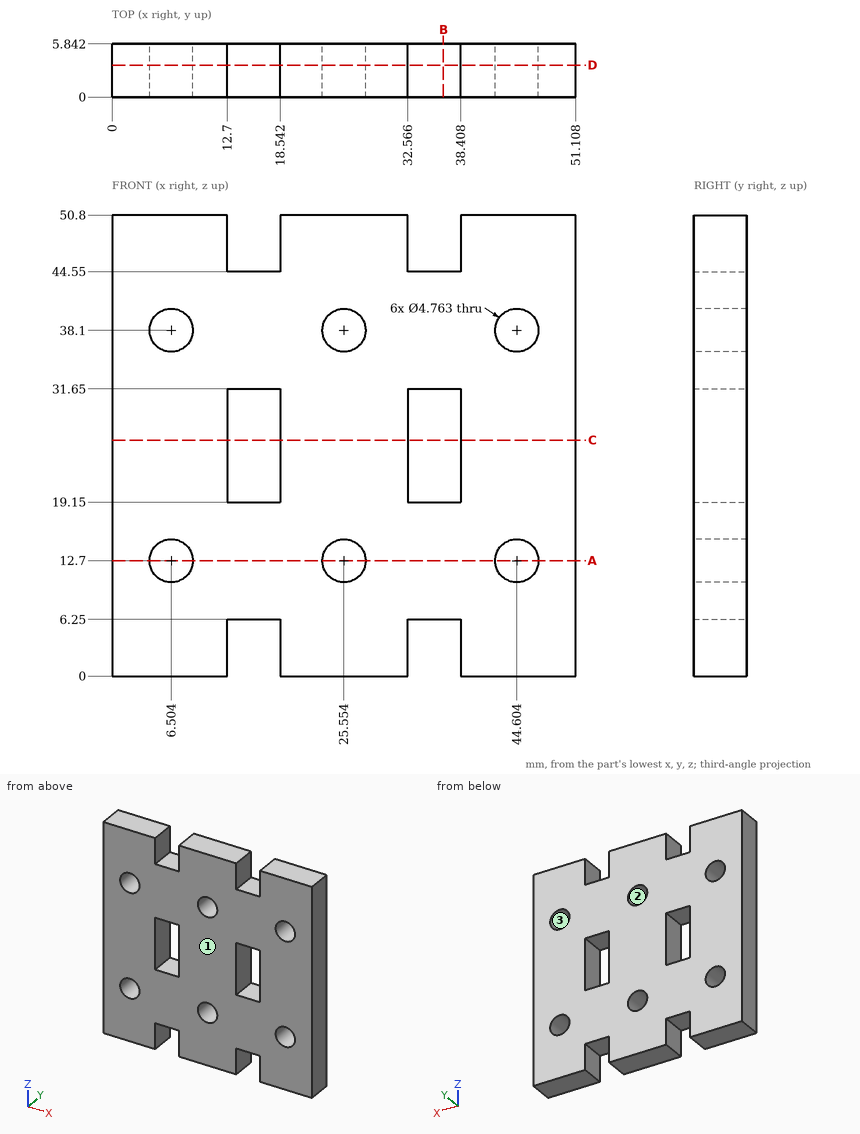
Study the drawing (mm; zero at the part's minimum x, y, z) and answer. Give positions to 0.01 mm unless a question says otherwise; leave off trailing zeros. Loops run counter-clockwise (first coordinate to the right, second up) from the corner with the lowest first, then second, coordinate; pieces in that order, holes last. Notation, with made-up numbers: (1, 57.25) - (34, 57.25) arc R10 cw to (34, 67.25) - close; hole circle Ø1 at (88.25, -15.75). An arc over 180 degrees is marked (long way). Answer as CSV lines item,"result". Start each with the question number.
1) Find section C-C (z = 26). Write down the section's boundary in (x, y) (1 decimal), then the cut area to 3 significant figures.
2) Straight lines are drawn through the part: L1, parallel to X at y = 2.3, z = 26.5 (1 decimal); L2, parallel to X at y = 4.2, z = 38.1 (1 decimal); L3, parallel to Z at x = 44.5, y = 2.4. For each, find the intervals that lie inside material, in ascending order. Write a range as from..to.
3) Determine the mould class of the marked faces 1, 2 and 3 for opening direction X: released by +X, released by -X, zero draft, split by the parting line, or undercut.
4) Each of these flat-tipped pins is pushed along its axis until it touches: pin 1 Ø2 at (x, y) = (37, 4.5) entering from +Z; pin 2 Ø2 at (x, z) = (14.5, 27.5) entering from +Y; pin 3 Ø1.8 at (x, y) = (15.5, 2.5) entering from -Z. Where does it stop, or does it pass through?
5) Find section B-B (x = 36.5). Write down the section's boundary in (y, z), then the cut area to 3 significant figures.
6) Find section D-D (y = 3.5). State how many separate pieces and enclosed holes the cut face has, then the cut area to 3 significant figures.
7) Find section A-A (z = 12.7). Write down the section's boundary in (x, y) (1 decimal), then the cut area to 3 significant figures.
Findings below:
1,outline,"(0, 0) - (12.7, 0) - (12.7, 5.8) - (0, 5.8) - close; (18.5, 0) - (32.6, 0) - (32.6, 5.8) - (18.5, 5.8) - close; (38.4, 0) - (51.1, 0) - (51.1, 5.8) - (38.4, 5.8) - close"
1,area,"230 mm^2"
2,L1,"0..12.7, 18.5..32.6, 38.4..51.1"
2,L2,"0..4.1, 8.9..23.2, 27.9..42.2, 47..51.1"
2,L3,"0..10.32, 15.08..35.72, 40.48..50.8"
3,face 1,"zero draft"
3,face 2,"undercut"
3,face 3,"undercut"
4,pin 1,"z = 44.55"
4,pin 2,"through"
4,pin 3,"z = 6.25"
5,outline,"(0, 6.25) - (5.84, 6.25) - (5.84, 19.15) - (0, 19.15) - close; (0, 31.65) - (5.84, 31.65) - (5.84, 44.55) - (0, 44.55) - close"
5,area,"151 mm^2"
6,separate pieces,"1"
6,enclosed holes,"8"
6,area,"2,200 mm^2"
7,outline,"(0, 0) - (4.1, 0) - (4.1, 5.8) - (0, 5.8) - close; (8.9, 0) - (23.2, 0) - (23.2, 5.8) - (8.9, 5.8) - close; (27.9, 0) - (42.2, 0) - (42.2, 5.8) - (27.9, 5.8) - close; (47, 0) - (51.1, 0) - (51.1, 5.8) - (47, 5.8) - close"
7,area,"215 mm^2"
